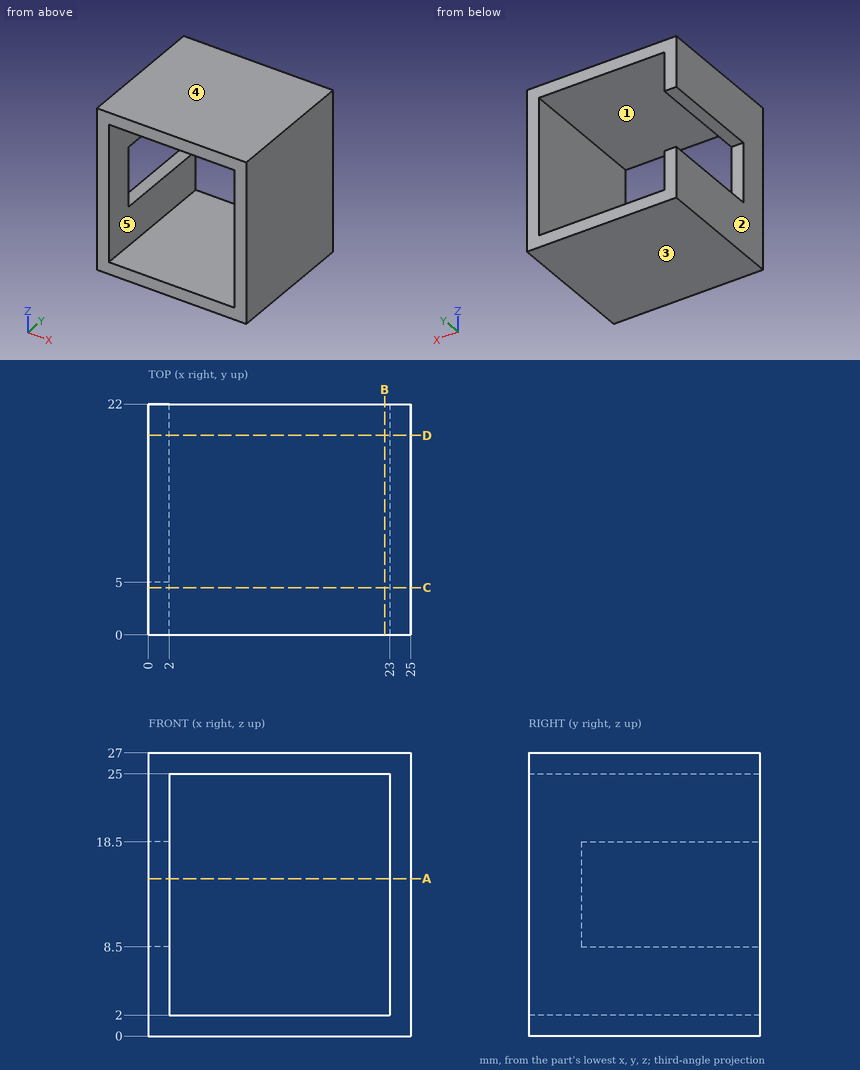
Here's the drawing with two shaded views (mm, measured from the low corner). I have some questions. A direction names the side the tool comes from. Coordinates: 2 decimals unless noted, no trailing zeros. Loops run counter-clockwise (first coordinate to the right, second up) from the corner with the lowest first, then second, coordinate; pieces in that order, holes last.
Item 1: Suppose I cut it at C-C (y = 4.5). Please give me the cut outline in (x, z).
Answers below:
outline: (0, 0) - (25, 0) - (25, 27) - (0, 27) - close; hole (2, 2) - (23, 2) - (23, 25) - (2, 25) - close
Item 2: Suppose I cut it at D-D (y = 19). Please give me the cut outline in (x, z).
Answers below:
outline: (0, 0) - (25, 0) - (25, 27) - (0, 27) - (0, 18.5) - (2, 18.5) - (2, 25) - (23, 25) - (23, 2) - (2, 2) - (2, 8.5) - (0, 8.5) - close
Item 3: Suppose I cut it at A-A (z = 15). Please give me the cut outline in (x, y).
Answers below:
outline: (0, 0) - (2, 0) - (2, 5) - (0, 5) - close; (23, 0) - (25, 0) - (25, 22) - (23, 22) - close
Item 4: I'm going to push a flat-ended pin straight in: pin 1 (0.6 mm diameter, centred on x = 0.5, z = 12, fed in from +Y). Where does the tip first touch, or does it pass through?
Answers below:
pin 1: stops at y = 5
Item 5: Suppose I cut it at B-B (x = 22.5). Please give me the cut outline in (y, z).
Answers below:
outline: (0, 0) - (22, 0) - (22, 2) - (0, 2) - close; (0, 25) - (22, 25) - (22, 27) - (0, 27) - close
Item 6: Which directions (+Z, -Z, +X, -X, +Y, -Y) give clear straight access to the entire face, cutting with the end or side of a thin tool? Please do the marked faces 4 and 5.
Answers below:
face 4: +Z, +X, -X, +Y, -Y
face 5: +Y, -Y
Item 7: If we mould it in two halves opening along X, with no side actions, what happens to the marked faces 1, 2 and 3? For each: released by +X, released by -X, zero draft, split by the parting line, or undercut.
Answers below:
face 1: undercut
face 2: released by -X
face 3: zero draft
Item 8: Please list where these lines run through material, in increasing order: L1, parallel to X at y = 18.5, z = 7.75; L2, parallel to Z at x = 15.25, y = 9.5; L3, parallel to X at y = 9.75, z = 12.
Answers below:
L1: x = 0 to 2, 23 to 25
L2: z = 0 to 2, 25 to 27
L3: x = 23 to 25
